Geometry: final body of the model. Coordinates: model frame, mm. Face numbers are marked on the shaded views. A direction names the side the tool comes from. Round coordinates to 2 decimals unless told otherwise and drop trailing zeros. Order: outer loops, then holes, each group sorted by start corner. A loop starts at its lowest first (then second) coordinate and runs counter-clockwise, first axis right, second up. Notation, with made-up numbers: (-0.5, 30.25) -> (23.5, 30.25) arc R7 ccw to (23.5, 41.25) -> close; hole circle Ø1 at (-6, -11). An arc over 180 degrees is marked (long way). Put each result on its own line as item: value.
```python
from build123d import *

# Parameters (mm, degrees)
SKETCH1_R           = 1.5
BOSS_EXTRUDE1_DEPTH = 5
FILLET2_R           = 3


with BuildPart() as part:
    # Sketch1 → Boss-Extrude1 (new body)
    with BuildSketch(Plane(origin=(0, 0, 0), x_dir=(1, 0, 0), z_dir=(0, 1, 0))):
        Polygon((0, 30), (0, 34), (30, 34), (30, 0), (0, 0), (0, 4), (26, 4), (26, 30), align=None)
        with Locations(Location((27, 2, 0), (0, 0, 270))):
            Circle(SKETCH1_R, mode=Mode.SUBTRACT)
        with Locations(Location((27, 32, 0), (0, 0, 270))):
            Circle(SKETCH1_R, mode=Mode.SUBTRACT)
        with Locations(Location((3, 32, 0), (0, 0, 270))):
            Circle(SKETCH1_R, mode=Mode.SUBTRACT)
        with Locations(Location((3, 2, 0), (0, 0, 270))):
            Circle(SKETCH1_R, mode=Mode.SUBTRACT)
    extrude(amount=BOSS_EXTRUDE1_DEPTH)

    # Fillet2
    # the kernel refuses this fillet: 3 mm, written as the material it adds along each edge
    with BuildSketch(Plane(origin=(26, 0, -30), x_dir=(0, 0, 1), z_dir=(0, 1, 0)), Plane(origin=(26, 0, -4), x_dir=(-1, 0, 0), z_dir=(0, 1, 0))) as fillet2_piece_1:
        with BuildLine():
            CenterArc((FILLET2_R, -FILLET2_R), FILLET2_R, 90, 90)
            Line((0, -FILLET2_R), (0, 0))
            Line((0, 0), (FILLET2_R, 0))
        make_face()
    extrude(amount=5)
    # the kernel refuses this fillet: 3 mm, written as the material it takes off along each edge
    with BuildSketch(Plane(origin=(30, -7.5, -34), x_dir=(-1, 0, 0), z_dir=(0, 1, 0)), Plane(origin=(0, -7.5, -34), x_dir=(0, 0, 1), z_dir=(0, 1, 0)), Plane(origin=(0, -7.5, -4), x_dir=(0, 0, 1), z_dir=(0, 1, 0)), Plane(origin=(0, -7.5, 0), x_dir=(1, 0, 0), z_dir=(0, 1, 0)), Plane(origin=(30, -7.5, 0), x_dir=(0, 0, -1), z_dir=(0, 1, 0))) as fillet2_2_piece_1:
        with BuildLine():
            CenterArc((FILLET2_R, FILLET2_R), FILLET2_R, 180, 90)
            Line((0, FILLET2_R), (0, 0))
            Line((0, 0), (FILLET2_R, 0))
        make_face()
    extrude(amount=20, mode=Mode.SUBTRACT)
    with BuildSketch(Plane(origin=(0, -7.5, -30), x_dir=(0, 0, -1), z_dir=(0, 1, 0))) as fillet2_2_piece_2:
        with BuildLine():
            CenterArc((FILLET2_R, -FILLET2_R), FILLET2_R, 90, 90)
            Line((0, -FILLET2_R), (0, 0))
            Line((0, 0), (FILLET2_R, 0))
        make_face()
    extrude(amount=20, mode=Mode.SUBTRACT)


solid = part.part
```
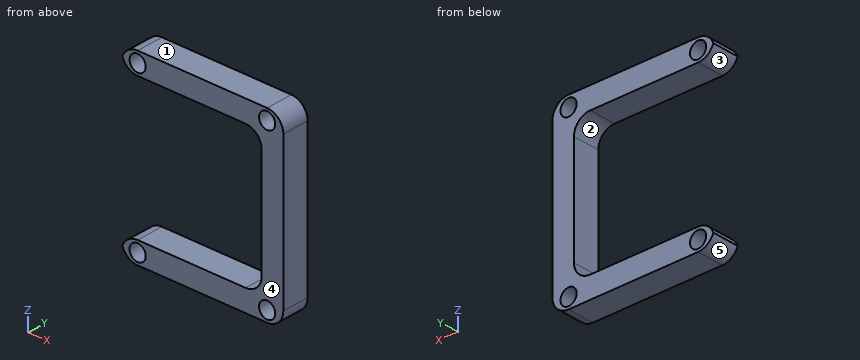
1. Contact query for flat-ended pins moving along their axis: P1, Ø3, axis at y = 3, z = -19, coming from the -X side; P2, Ø2.5, axis at x = 3, z = -2, coming from the +Y side. Output: stop coordinate, or through.
Ans:
P1: x = 26
P2: through
2. Cut plane D-D on z = -25. Return loops of the section in (x, y), and give its area (3 significant figures).
Ans:
outline: (26, 0) -> (30, 0) -> (30, 5) -> (26, 5) -> close
area: 20.0 mm²
3. Draft query along Z for the marked faces 3, 4 and 5. Return one class per face: +Z half, -Z half, draft (parallel to the pull), parting line (faces both ways), or undercut.
Ans:
face 3: undercut
face 4: draft
face 5: -Z half
4. Material intervals for probe 1 along X at (y, z) = (2.15, -32); probe 2 along Z at (x, y) = (3.5, 4.55); probe 3 along Z at (x, y) = (18.25, 1.95), sorted ascending.
Ans:
probe 1: 0.17 to 1.5, 4.5 to 25.5, 28.5 to 29.83
probe 2: -34 to -33.41, -30.59 to -30, -4 to -3.41, -0.59 to 0
probe 3: -34 to -30, -4 to 0
5. Cut plane A-A on x = 15. Return loops of the section in (y, z).
Ans:
outline: (0, -34) -> (5, -34) -> (5, -30) -> (0, -30) -> close; (0, -4) -> (5, -4) -> (5, 0) -> (0, 0) -> close
6. Cut plane B-B on y = 2.6. Return loops of the section in (x, z).
Ans:
outline: (0.17, -32) arc R3 ccw to (3, -34) -> (27, -34) arc R3 ccw to (30, -31) -> (30, -3) arc R3 ccw to (27, 0) -> (3, 0) arc R3 ccw to (0.17, -2) arc R3 ccw to (3, -4) -> (23, -4) arc R3 cw to (26, -7) -> (26, -27) arc R3 cw to (23, -30) -> (3, -30) arc R3 ccw to start; hole circle Ø3 at (3, -32); hole circle Ø3 at (3, -2); hole circle Ø3 at (27, -32); hole circle Ø3 at (27, -2)
7. Cut plane C-C on x = 2. Return loops of the section in (y, z), and give its area (3 significant figures).
Ans:
outline: (0, -33.83) -> (5, -33.83) -> (5, -33.12) -> (0, -33.12) -> close; (0, -30.88) -> (5, -30.88) -> (5, -30.17) -> (0, -30.17) -> close; (0, -3.83) -> (5, -3.83) -> (5, -3.12) -> (0, -3.12) -> close; (0, -0.88) -> (5, -0.88) -> (5, -0.17) -> (0, -0.17) -> close
area: 14.2 mm²
8. Set-up query: the marked faces 1 and 2. Return all of +Z, -Z, +X, -X, +Y, -Y with unobstructed straight access to the full face (end or side cutting, diameter ignored); none if empty.
Ans:
face 1: +Z, +X, -X, +Y, -Y
face 2: -X, +Y, -Y
